```python
from build123d import *

# Parameters (mm, degrees)
SKETCH1_R             = 1.6
BOSS_EXTRUDE1_DEPTH   = 2
BOSS_EXTRUDE1_2_DEPTH = 2
SKETCH1_5_R           = 10
SKETCH1_5_R_2         = 6.5
BOSS_EXTRUDE2_DEPTH   = 7
SKETCH1_6_R           = 6.5
SKETCH1_6_R_2         = 3
BOSS_EXTRUDE3_DEPTH   = 2


with BuildPart() as part:
    # Sketch1 → Boss-Extrude1 (new body)
    with BuildSketch(Plane(origin=(0, 0, 0), x_dir=(0, 0, -1), z_dir=(1, 0, 0))):
        with BuildLine():
            Line((-3.333333333, 9.428090416), (-16.666666667, 4.714045208))
            ThreePointArc((-16.666666667, 4.714045208), (-20, 0), (-16.666666667, -4.714045208))
            Line((-16.666666667, -4.714045208), (-3.333333333, -9.428090416))
            ThreePointArc((-3.333333333, -9.428090416), (-10, 0), (-3.333333333, 9.428090416))
        make_face()
        with Locations((-15, 0)):
            Circle(SKETCH1_R, mode=Mode.SUBTRACT)
    extrude(amount=BOSS_EXTRUDE1_DEPTH)



with BuildPart() as body_2:
    # Sketch1 → Boss-Extrude1 2 (new body)
    with BuildSketch(Plane(origin=(0, 0, 0), x_dir=(0, 0, -1), z_dir=(1, 0, 0))):
        with BuildLine():
            Line((16.666666667, 4.714045208), (3.333333333, 9.428090416))
            ThreePointArc((3.333333333, 9.428090416), (8.164965809, 5.773502692), (10, 0))
            ThreePointArc((10, 0), (8.164965809, -5.773502692), (3.333333333, -9.428090416))
            Line((3.333333333, -9.428090416), (16.666666667, -4.714045208))
            ThreePointArc((16.666666667, -4.714045208), (20, 0), (16.666666667, 4.714045208))
        make_face()
        with Locations((15, 0)):
            Circle(SKETCH1_R, mode=Mode.SUBTRACT)
    extrude(amount=BOSS_EXTRUDE1_2_DEPTH)


with BuildPart() as part_1:
    add(part.part)

    add(body_2.part)  # Boss-Extrude2 merges body 2
    # Sketch1<5> → Boss-Extrude2 (add)
    with BuildSketch(Plane(origin=(0, 0, 0), x_dir=(0, 0, -1), z_dir=(1, 0, 0))):
        Circle(SKETCH1_5_R)
        Circle(SKETCH1_5_R_2, mode=Mode.SUBTRACT)
    extrude(amount=BOSS_EXTRUDE2_DEPTH)

    # Sketch1<6> → Boss-Extrude3 (add)
    with BuildSketch(Plane(origin=(0, 0, 0), x_dir=(0, 0, -1), z_dir=(1, 0, 0))):
        Circle(SKETCH1_6_R)
        Circle(SKETCH1_6_R_2, mode=Mode.SUBTRACT)
    extrude(amount=BOSS_EXTRUDE3_DEPTH)


solid = part_1.part
```
The model under review builds one solid part; all positions refer to its coordinate system, in mm. A direction names the side the tool comes from. Round coordinates to 2 decimals unless told otherwise and drop trailing zeros. Loops run counter-clockwise (first coordinate to the right, second up) from the corner with the lowest first, then second, coordinate; pieces in that order, holes last. Notation, with made-up numbers: (28.5, 27) -> (34.5, 27) arc R31 cw to (34.5, 64) -> close; hole circle Ø9 at (-3.5, 32.5). An arc over 180 degrees is marked (long way). Answer as a JSON object with one key per item and string values. Group by question number.
1) For faces 1 (the face through (2, 0, 12)), 2 (the face through (0, 0, -4)), 3 (the face through (2, -1, -3)), list the 3-axis set-ups (+Z, -Z, +X, -X, +Y, -Y) from which the entire face can be reached by the end or side of a thin tool; tool diameter is ignored.
2) We need section C-C on x = 1.5. Write out the cut boundary in (y, z).
3) We need section B-B on y = 0. Write out the cut boundary in (x, z), then the cut area to 3 significant figures.
4) For pin 1 Ø1.9 at (y, z) = (0, -15) entering from +X; pin 2 Ø4 at (x, y) = (5, -6) entering from -Z; pin 3 Ø1 at (x, z) = (2, -14.5) entering from -Y, all flat-tipped, find the tip position at first contact; note any pin that passes through.
5) Mouldability with a two-part tool opening along Z and no side actions: class faces 4 (the face through (4.465, -3.955, 5.158)), 5 (the face through (0.99, 0.07, -13.4)), 6 (the face through (1, 0, -20)), 7 (the face through (0.986, 7.104, 9.907)) as released by +Z, released by -Z, zero draft, split by the parting line, or undercut.
6) For line 1 (Y direction, x = 4.65, z = 0); line 2 (Z direction, x = 4.75, y = -2.5); line 3 (X direction, y = -1.5, z = 14), list the stretches that pass through material, from the lowest coordinate up. Write a range as [from, to].
7) We need section D-D on y = 3.75. Write out the cut boundary in (x, z).
8) We need section A-A on z = 0. Write out the cut boundary in (x, y), then the cut area to 3 significant figures.
Result set:
{
 "1": {"face 1": "+Z, +X", "face 2": "+Z, -Z, -X, +Y, -Y", "face 3": "+X"},
 "2": {"outline": "(-9.43, -3.33) -> (-4.71, -16.67) arc R5 ccw to (4.71, -16.67) -> (9.43, -3.33) arc R10 ccw to (9.43, 3.33) -> (4.71, 16.67) arc R5 ccw to (-4.71, 16.67) -> (-9.43, 3.33) arc R10 ccw to start; hole circle Ø6 at (0, 0); hole circle Ø3.2 at (0, -15); hole circle Ø3.2 at (0, 15)"},
 "3": {"outline": "(0, -20) -> (2, -20) -> (2, -16.6) -> (0, -16.6) -> close; (0, -13.4) -> (2, -13.4) -> (2, -10) -> (7, -10) -> (7, -6.5) -> (2, -6.5) -> (2, -3) -> (0, -3) -> close; (0, 3) -> (2, 3) -> (2, 6.5) -> (7, 6.5) -> (7, 10) -> (2, 10) -> (2, 13.4) -> (0, 13.4) -> close; (0, 16.6) -> (2, 16.6) -> (2, 20) -> (0, 20) -> close", "area": "90.2 mm²"},
 "4": {"pin 1": "through", "pin 2": "z = -9.17", "pin 3": "y = -5.66"},
 "5": {"face 4": "undercut", "face 5": "undercut", "face 6": "released by -Z", "face 7": "released by +Z"},
 "6": {"line 1": "[-10, -6.5], [6.5, 10]", "line 2": "[-9.68, -6], [6, 9.68]", "line 3": "[0, 2]"},
 "7": {"outline": "(0, -18.31) -> (2, -18.31) -> (2, -9.27) -> (7, -9.27) -> (7, -5.31) -> (2, -5.31) -> (2, 5.31) -> (7, 5.31) -> (7, 9.27) -> (2, 9.27) -> (2, 18.31) -> (0, 18.31) -> close"},
 "8": {"outline": "(0, -10) -> (7, -10) -> (7, -6.5) -> (2, -6.5) -> (2, -3) -> (0, -3) -> close; (0, 3) -> (2, 3) -> (2, 6.5) -> (7, 6.5) -> (7, 10) -> (0, 10) -> close", "area": "63.0 mm²"}
}
